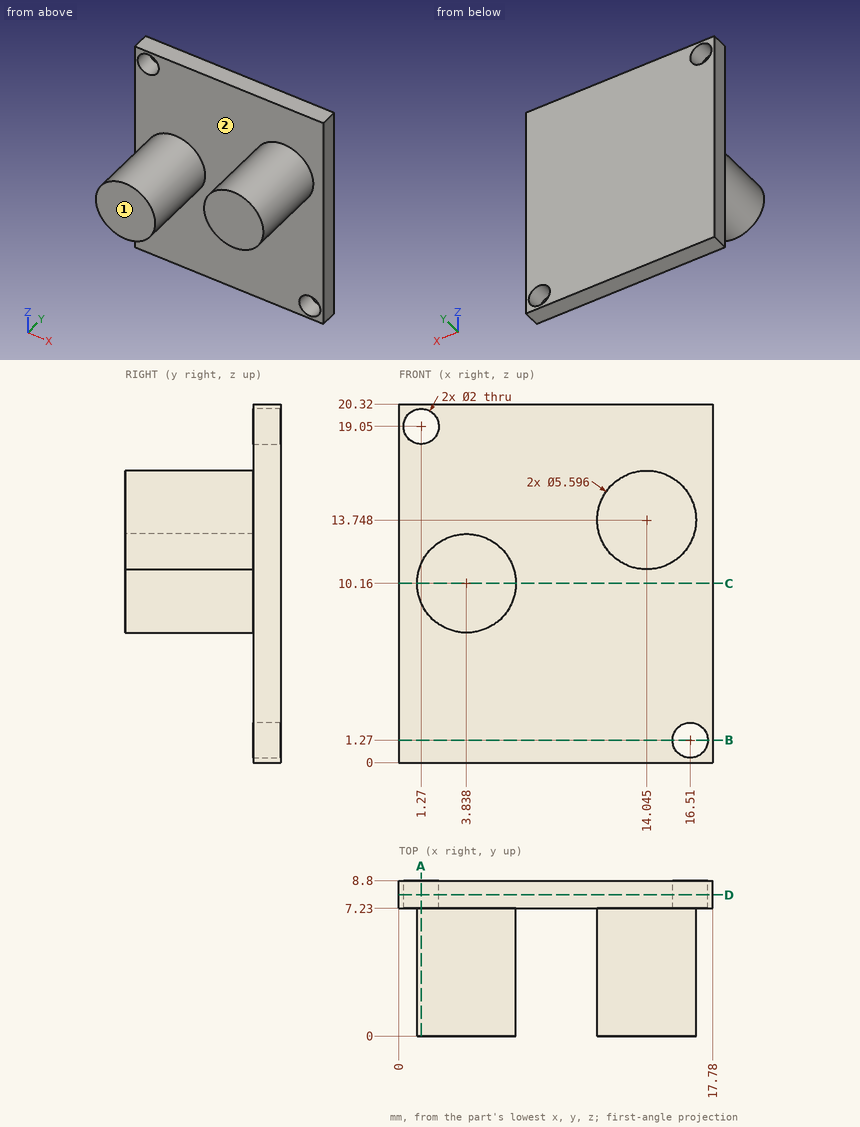
Design review of the part shown in the three views and the two pictorial views. Dimensions are in mm from the part's minimum x, y and z. A direction names the side the tool comes from. Round coordinates to 2 decimals unless told otherwise and drop trailing zeros. Loops run counter-clockwise (first coordinate to the right, second up) from the corner with the lowest first, then second, coordinate; pieces in that order, holes last. Notation, with made-up numbers: (87, 63) -> (111, 63) arc R10 ccw to (111, 80) -> close; hole circle Ø1 at (-34, -7). An arc over 180 degrees is marked (long way). Return JSON: item names as keys, results as strings.
(1) Add section D-D on y = 8. Write out the cut boundary in (x, z).
Solved:
{"outline": "(0, 0) -> (17.78, 0) -> (17.78, 20.32) -> (0, 20.32) -> close; hole circle Ø2 at (1.27, 19.05); hole circle Ø2 at (16.51, 1.27)"}
(2) For line 1 (X direction, y = 8.45, z = 19.05); line 2 (X direction, y = 7.65, z = 1.27); line 3 (Y direction, x = 7.75, z = 13), list the stretches that pass through material, from the lowest coordinate up.
Solved:
{"line 1": "0 to 0.27, 2.27 to 17.78", "line 2": "0 to 15.51, 17.51 to 17.78", "line 3": "7.23 to 8.8"}
(3) For pin 1 (5 mm diameter, centred on x = 7.5, y = 4, fed in from -Z) (1 decimal); pin 2 (3 mm diameter, centred on x = 4.5, y = 3, fed in from +Z), all flat-tipped, find the tip position at first contact; note any pin that passes through.
Solved:
{"pin 1": "z = 7.6", "pin 2": "z = 12.96"}
(4) For the marked faces 1 and 2, list the 3-axis set-ups (+Z, -Z, +X, -X, +Y, -Y) from which the entire face can be reached by the end or side of a thin tool; tool diameter is ignored.
Solved:
{"face 1": "+Z, -Z, +X, -X, -Y", "face 2": "-Y"}
(5) Add section A-A on x = 1.27. Write out the cut boundary in (y, z).
Solved:
{"outline": "(0, 9.05) -> (7.23, 9.05) -> (7.23, 0) -> (8.8, 0) -> (8.8, 18.05) -> (7.23, 18.05) -> (7.23, 11.27) -> (0, 11.27) -> close; (7.23, 20.05) -> (8.8, 20.05) -> (8.8, 20.32) -> (7.23, 20.32) -> close"}
(6) Add section B-B on z = 1.27. Write out the cut boundary in (x, y).
Solved:
{"outline": "(0, 7.23) -> (15.51, 7.23) -> (15.51, 8.8) -> (0, 8.8) -> close; (17.51, 7.23) -> (17.78, 7.23) -> (17.78, 8.8) -> (17.51, 8.8) -> close"}
(7) Add section C-C on z = 10.16. Write out the cut boundary in (x, y).
Solved:
{"outline": "(0, 7.23) -> (1.04, 7.23) -> (1.04, 0) -> (6.64, 0) -> (6.64, 7.23) -> (17.78, 7.23) -> (17.78, 8.8) -> (0, 8.8) -> close"}
